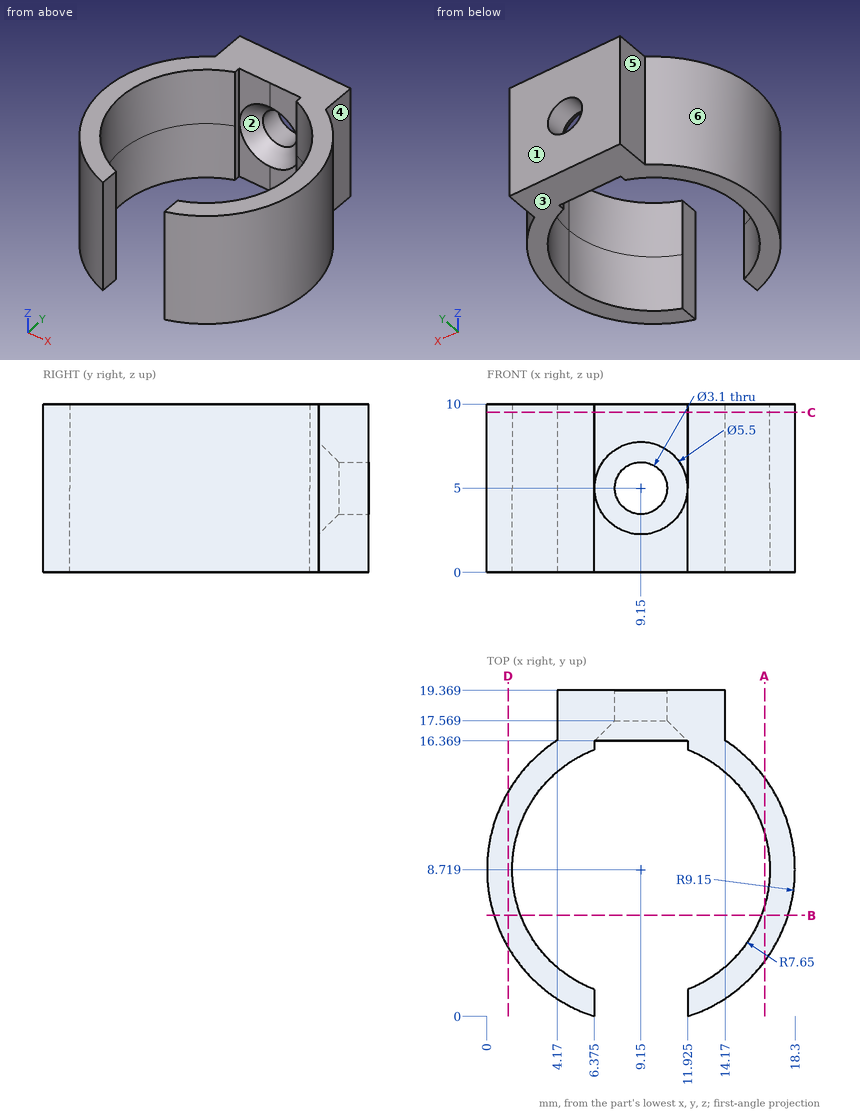
Answer from the drawing. Dimensions are ordinates in mm from the lowest x, y and z of the part. A direction names the side the tool comes from. Give positions to 0.01 mm unless a question says otherwise; leave off trailing zeros. Loops run counter-clockwise (first coordinate to the right, second up) from the corner with the lowest first, then second, coordinate; pieces in that order, holes last. Notation, with made-up numbers: (64.25, 10.25) -> (89.25, 10.25) arc R28 ccw to (89.25, 32.25) -> close; hole circle Ø11 at (54, 3). An arc over 180 degrees is marked (long way). Answer as CSV lines item,"result".
Item 1: Consider line 1 (Z direction, x = 9.15, y = 18.2); line 2 (X direction, y = 18.3, z = 5); line 3 (Y direction, x = 9.25, z = 9.25). Determine where each line is inside the solid, lowest interval first. Write a range as [from, to].
Returned:
line 1,"z = [0, 3.45], [6.55, 10]"
line 2,"x = [4.17, 7.6], [10.7, 14.17]"
line 3,"y = [16.37, 19.37]"
Item 2: Find section D-D on x = 1.25. Give the vertices of the cut face in (y, z).
Returned:
outline,"(4.1, 0) -> (13.34, 0) -> (13.34, 10) -> (4.1, 10) -> close"
Item 3: For the marked faces 4, 5 and 6, determine the directions among +Z, -Z, +X, -X, +Y, -Y from which every point of the face is accessible in a straight line to the end or side of a thin tool.
Returned:
face 4,"+Z, -Z, +X, +Y"
face 5,"+Z, -Z, -X, +Y"
face 6,"+Z, -Z, -X"
Item 4: Find section C-C on z = 9.5. Give the vertices of the cut face in (x, y) (3 decimals), plus the area to 3 significant figures.
Returned:
outline,"(4.17, 16.395) arc R9.15 ccw to (6.375, 0) -> (6.375, 1.59) arc R7.65 cw to (6.375, 15.848) -> (6.375, 16.369) -> (11.925, 16.369) -> (11.925, 15.848) arc R7.65 cw to (11.925, 1.59) -> (11.925, 0) arc R9.15 ccw to (14.17, 16.369) -> (14.17, 19.369) -> (4.17, 19.369) -> close"
area,"89.5 mm²"
Item 5: Find section B-B on y = 6. Give the vertices of the cut face in (x, z).
Returned:
outline,"(0.41, 0) -> (2, 0) -> (2, 10) -> (0.41, 10) -> close; (16.3, 0) -> (17.89, 0) -> (17.89, 10) -> (16.3, 10) -> close"
Item 6: Each of these flat-tipped pins is pushed along its axis until it touches: pin 1 (0.5 mm diameter, centred on y = 1, z = 3.5, fed in from +X); pin 2 (0.9 mm diameter, centred on y = 18, z = 4, fed in from -X); pin 3 (2 mm diameter, centred on x = 11, z = 3, fed in from -Y). Where does it stop, or does it pass through?
Returned:
pin 1,"stops at x = 14.44"
pin 2,"stops at x = 4.17"
pin 3,"stops at y = 0"
Item 7: Find section A-A on x = 16.5. Give the vertices of the cut face in (y, z).
Returned:
outline,"(3.27, 0) -> (6.6, 0) -> (6.6, 10) -> (3.27, 10) -> close; (10.84, 0) -> (14.17, 0) -> (14.17, 10) -> (10.84, 10) -> close"
Item 8: Determine the mould class of the marked faces 1, 2 and 3 for opening direction Z: +Z half, -Z half, draft (parallel to the pull), parting line (faces both ways), or undercut.
Returned:
face 1,"draft"
face 2,"undercut"
face 3,"-Z half"
